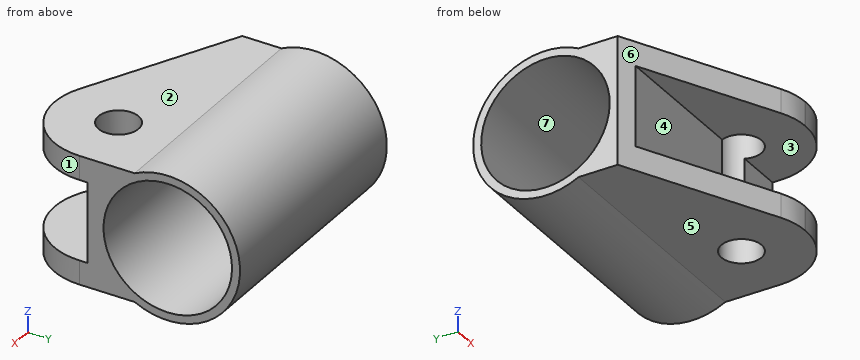
from build123d import *

# Parameters (mm, degrees)
SKETCH1_R                       = 9
SKETCH1_R_2                     = 8
BOSS_EXTRUDE1_DEPTH             = 30
SKETCH2_W                       = 30
SKETCH2_H                       = 16
BOSS_EXTRUDE2_DEPTH             = 10
BOSS_EXTRUDE2_DIRECTION_2_REACH = 38.125
CUT_EXTRUDE1_DEPTH              = 40.37003937
SKETCH4_W                       = 10
SKETCH4_H                       = 9
CUT_EXTRUDE2_DEPTH              = 37.633318168
FILLET1_R                       = 8
SKETCH5_R                       = 2.5
CUT_EXTRUDE3_DEPTH              = 40.37003937


with BuildPart() as part:
    # Sketch1 → Boss-Extrude1 (new body)
    with BuildSketch(Plane(origin=(0, 0, 0), x_dir=(0, 0, -1), z_dir=(1, 0, 0))):
        Circle(SKETCH1_R)
        Circle(SKETCH1_R_2, mode=Mode.SUBTRACT)
    extrude(amount=BOSS_EXTRUDE1_DEPTH)

    # Sketch2 → Boss-Extrude2 (add)
    with BuildSketch(Plane(origin=(0, -9, 0), x_dir=(-1, 0, 0), z_dir=(0, -1, 0))):
        with Locations((-15, 0)):
            Rectangle(SKETCH2_W, SKETCH2_H)
    extrude(amount=BOSS_EXTRUDE2_DEPTH)

    # Sketch2 → Boss-Extrude2 direction 2 (add, up to next)
    with BuildSketch(Plane(origin=(0, -9, 0), x_dir=(-1, 0, 0), z_dir=(0, -1, 0)), mode=Mode.PRIVATE) as boss_extrude2_direction_2_sk1:
        with Locations((-15, 0)):
            Rectangle(SKETCH2_W, SKETCH2_H)
    boss_extrude2_direction_2_tool1 = extrude(boss_extrude2_direction_2_sk1.sketch, amount=-BOSS_EXTRUDE2_DIRECTION_2_REACH, mode=Mode.PRIVATE) - part.part
    add(boss_extrude2_direction_2_tool1.solids().sort_by_distance((15, -9, 0))[0])
    add(boss_extrude2_direction_2_tool1.solids().sort_by_distance((15, -9, 0))[1])

    # Sketch3 → Cut-Extrude1 (cut, through all)
    with BuildSketch(Plane.XY.offset(8)):
        Polygon((0, -19), (0, -9), (20, -19), align=None)
    extrude(amount=-CUT_EXTRUDE1_DEPTH, mode=Mode.SUBTRACT)

    # Sketch4 → Cut-Extrude2 (cut, through all)
    with BuildSketch(Plane(origin=(30, 0, 0), x_dir=(0, 0, -1), z_dir=(1, 0, 0))):
        with Locations((0, -14.5)):
            Rectangle(SKETCH4_W, SKETCH4_H)
    extrude(amount=-CUT_EXTRUDE2_DEPTH, mode=Mode.SUBTRACT)

    # Fillet1
    fillet1_edges = [part.edges().sort_by_distance(p)[0] for p in [
        (30, -19, -6.5),
        (20, -19, -6.5),
        (20, -19, 6.5),
        (30, -19, 6.5),
    ]]
    fillet(fillet1_edges, radius=FILLET1_R)

    # Sketch5 → Cut-Extrude3 (cut, through all)
    with BuildSketch(Plane.XY.offset(8)):
        with Locations((22, -11)):
            Circle(SKETCH5_R)
    extrude(amount=-CUT_EXTRUDE3_DEPTH, mode=Mode.SUBTRACT)


solid = part.part
Part model, mm, in its own coordinate system. Face numbers are marked on the shaded views. A direction names the side the tool comes from. Coordinates: 2 decimals unless noted, no trailing zeros. Loops run counter-clockwise (first coordinate to the right, second up) from the corner with the lowest first, then second, coordinate; pieces in that order, holes last. Notation, with made-up numbers: (-26.75, -36) -> (-0.75, -36) arc R14 ccw to (-0.75, -17) -> close; hole circle Ø1 at (15, 21). An arc over 180 degrees is marked (long way). Use a Markdown table: item, result. Add a question column.
Item 1: Band-saw the part on B-B on y = 0. Write the cut outline in (x, z).
Item 2: Band-saw the part on D-D on z = 6.5. Write the cut outline in (x, y), plus the area to 3 significant figures.
Item 3: Band-saw the part on A-A on z = 0. Write the cut outline in (x, y), plus the area to 3 significant figures.
Item 4: Probe probe 1 along Y at (x, z) = (20.5, 0); probe 2 along Y at (x, z) = (22.75, 7); probe 3 along Y at (x, z) = (18.5, 0). List the from-to ranges inside material, lowest first.
Item 5: Flat gauge pins, fed straight in: P1, Ø10, axis at x = 11, y = -11, coming from the +Z side; P2, Ø5, axis at x = 25.5, z = 0.5, coming from the -Y side; P3, Ø10, axis at x = 14.5, y = -14, coming from the -Z side; P4, Ø8, axis at x = 10, y = -4, coming from the +Z side. Where does each tip first touch, or does it go through?
Item 6: Which spindle directions (+Z, -Z, +X, -X, +Y, -Y) get a long thin tool onto all of the face, cutting with end or side? Do the marked faces 1, 2 and 3. Say none if no direction does.
Item 7: Pull direction Z, two halves, no side cores. Call the marked faces 4, 5, 6 and 7: +Z half, -Z half, draft (parallel to the pull), parting line (faces both ways), or undercut.
Item 8: Band-saw the part on C-C on x = 11.5. Write the cut outline in (y, z).
Geometry says:
| question | item | result |
|---|---|---|
| 1 | outline | (0, -9) -> (30, -9) -> (30, -8) -> (0, -8) -> close; (0, 8) -> (30, 8) -> (30, 9) -> (0, 9) -> close |
| 2 | outline | (0, -9) -> (18.31, -18.16) arc R8 ccw to (21.89, -19) -> (22, -19) arc R8 ccw to (30, -11) -> (30, -4.66) -> (0, -4.66) -> close; (0, 4.66) -> (30, 4.66) -> (30, 6.22) -> (0, 6.22) -> close; hole circle Ø5 at (22, -11) |
| 2 | area | 343 mm² |
| 3 | outline | (0, -9) -> (2, -10) -> (19.71, -10) arc R2.5 cw to (24.29, -10) -> (30, -10) -> (30, -8) -> (0, -8) -> close; (0, 8) -> (30, 8) -> (30, 9) -> (0, 9) -> close |
| 3 | area | 84.0 mm² |
| 4 | probe 1 | -9 to -8, 8 to 9 |
| 4 | probe 2 | -18.96 to -13.38, -8.62 to -3.87, 3.87 to 5.66 |
| 4 | probe 3 | -10 to -8, 8 to 9 |
| 5 | P1 | z = 8 |
| 5 | P2 | y = -10 |
| 5 | P3 | z = -8 |
| 5 | P4 | z = 9 |
| 6 | face 1 | +Z, -Z, +X, -Y |
| 6 | face 2 | +Z, +X, -X, -Y |
| 6 | face 3 | +X, -X, -Y |
| 7 | face 4 | undercut |
| 7 | face 5 | -Z half |
| 7 | face 6 | draft |
| 7 | face 7 | undercut |
| 8 | outline | (-14.75, -8) -> (-4.12, -8) arc R9 ccw (long way) to (-4.12, 8) -> (-14.75, 8) -> (-14.75, 5) -> (-10, 5) -> (-10, -5) -> (-14.75, -5) -> close; hole circle Ø16 at (0, 0) |
